Geometry: see drawing. Coordinates: mm, zero at the bounding-box minimum. Round coordinates to 2 decimals unless told otherwise and drop trailing zeros. Order: outer loops, then holes, each group sorted by start corner. A loop starts at its lowest first (then second) coordinate and runs counter-clockwise, first axis right, second up. Notation, with made-up numbers: (80.5, -32) - (107.5, -32) arc R27 cw to (107.5, -4) - close; hole circle Ø10 at (-16, 39). An arc over 180 degrees is marked (long way). Put each result on its own line as item: value. Start each with the question number.
1) Section D-D on y = 9.5. Output: boundary loops of the cut face in (x, z), then the cut area to 3 significant figures.
2) Line query: probe 1 along Y at (x, z) = (10, 2); probe 2 along Y at (x, z) = (72.5, 1.3); probe 3 along X at (y, z) = (23.25, 5.75). Output: solid intervals per line, ascending. Write a range as [from, to].
3) Section A-A on x = 47.5. Output: boundary loops of the cut face in (y, z), then the cut area to 3 significant figures.
4) Section C-C on x = 160. Output: boundary loops of the cut face in (y, z).
5) Contact query for flat-ended pins moving along their axis: P1, Ø1.9, axis at x = 160, y = 15, coming from the -Z side; P2, Ø10.5, axis at x = 97.5, y = 15, coming from the +Z side. Output: stop coordinate, or through.
6) Section B-B on z = 1.5. Output: boundary loops of the cut face in (x, y), then the cut area to 3 significant figures.
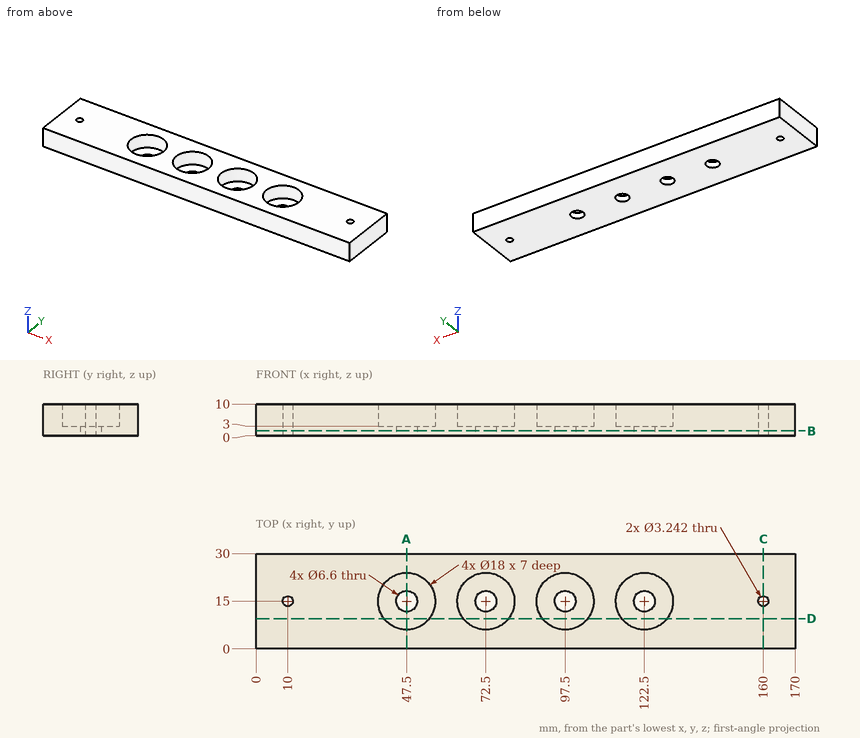
Answer sheet:
1. outline: (0, 0) - (170, 0) - (170, 10) - (129.62, 10) - (129.62, 3) - (115.38, 3) - (115.38, 10) - (104.62, 10) - (104.62, 3) - (90.38, 3) - (90.38, 10) - (79.62, 10) - (79.62, 3) - (65.38, 3) - (65.38, 10) - (54.62, 10) - (54.62, 3) - (40.38, 3) - (40.38, 10) - (0, 10) - close
1. area: 1,300 mm^2
2. probe 1: [0, 13.38], [16.62, 30]
2. probe 2: [0, 11.7], [18.3, 30]
2. probe 3: [0, 43.9], [51.1, 68.9], [76.1, 93.9], [101.1, 118.9], [126.1, 170]
3. outline: (0, 0) - (11.7, 0) - (11.7, 3) - (6, 3) - (6, 10) - (0, 10) - close; (18.3, 0) - (30, 0) - (30, 10) - (24, 10) - (24, 3) - (18.3, 3) - close
3. area: 154 mm^2
4. outline: (0, 0) - (13.38, 0) - (13.38, 10) - (0, 10) - close; (16.62, 0) - (30, 0) - (30, 10) - (16.62, 10) - close
5. P1: through
5. P2: z = 3
6. outline: (0, 0) - (170, 0) - (170, 30) - (0, 30) - close; hole circle Ø3.24 at (10, 15); hole circle Ø6.6 at (47.5, 15); hole circle Ø6.6 at (72.5, 15); hole circle Ø6.6 at (97.5, 15); hole circle Ø6.6 at (122.5, 15); hole circle Ø3.24 at (160, 15)
6. area: 4,950 mm^2
